from build123d import *

# Parameters (mm, degrees)
SKETCH_1_W         = 66.15
SKETCH_1_H         = 48
EXTRUDE_1_DEPTH    = 6
HOLE_WIZARD_M3_2_D = 2.5
HOLE_WIZARD_M3_3_D = 2.5


with BuildPart() as part:
    # 草图1 → 凸台-拉伸1 (new body)
    with BuildSketch(Plane.XY):
        Rectangle(SKETCH_1_W, SKETCH_1_H)
    extrude(amount=EXTRUDE_1_DEPTH)

    # M3 螺纹孔2 (through all)
    with Locations(Plane.ZY.offset(33.075)):
        with Locations((3, 12), (3, -12), (3, 0)):
            Hole(HOLE_WIZARD_M3_2_D / 2)

    # M3 螺纹孔3 (through all)
    with Locations(Plane(origin=(0, 24, 0), x_dir=(1, 0, 0), z_dir=(0, 1, 0))):
        with Locations((0, -3), (20, -3), (-20, -3)):
            Hole(HOLE_WIZARD_M3_3_D / 2)


solid = part.part
Source: CAD feature listing. Evaluate the final solid. Frame: model axes, mm. Round coordinates to 2 decimals unless told otherwise and drop trailing zeros. Loops run counter-clockwise (first coordinate to the right, second up) from the corner with the lowest first, then second, coordinate; pieces in that order, holes last. Notation, with made-up numbers: (-9.75, -25.5) -> (33.25, -25.5) arc R12 ccw to (33.25, -20.5) -> close; hole circle Ø1 at (83, 75). An arc over 180 degrees is marked (long way). Answer as a JSON object with one key per item and string values. Group by question number.
Q1. Section query B-B (y = -19). Output: boundary loops of the cut face in (x, z) (3 decimals).
Q2. Contact query for a flat-ended pin moving along its axis: P1, Ø3, axis at x = 20, z = 3, coming from the +Y side. Output: stop coordinate, or through.
Q3. Ray query, line 1 (X direction, y = 19.5, z = 3.15) (3 decimals); line 2 (Y direction, x = 12.75, z = 3); line 3 (Z direction, x = -5.75, y = -12). Return the intervals inside material, ascending. Write a range as from..to.
Q4. Mould query, pull axis Z, two halves, no side actions, for faces 1 (the cylindrical face through (10.14, 12.05, 4.25)), 2 (the flat face through (0, 0, 0)), 3 (the cylindrical face through (19.423, 5.916, 4.109)), 4 (the flat face through (33.075, -0.3, 1.6)). Classes: pulls with the +Z half, pulls with the -Z half, needs draft (parallel to the pull), parting line crosses it, or undercut.
Q5. Section query A-A (x = 7). Output: boundary loops of the cut face in (y, z).
Completed:
{
 "1": {"outline": "(-33.075, 0) -> (33.075, 0) -> (33.075, 6) -> (-33.075, 6) -> close; hole circle Ø2.5 at (-20, 3); hole circle Ø2.5 at (0, 3); hole circle Ø2.5 at (20, 3)"},
 "2": {"P1": "y = 24"},
 "3": {"line 1": "-33.075..-21.241, -18.759..-1.241, 1.241..18.759, 21.241..33.075", "line 2": "-24..-13.25, -10.75..-1.25, 1.25..10.75, 13.25..24", "line 3": "0..1.75, 4.25..6"},
 "4": {"face 1": "undercut", "face 2": "pulls with the -Z half", "face 3": "undercut", "face 4": "needs draft"},
 "5": {"outline": "(-24, 0) -> (24, 0) -> (24, 6) -> (-24, 6) -> close; hole circle Ø2.5 at (-12, 3); hole circle Ø2.5 at (0, 3); hole circle Ø2.5 at (12, 3)"}
}
